from build123d import *

# Parameters (mm, degrees)
F1_DEPTH = 23
F2_DEPTH = 23
F3_DEPTH = 10
F4_R     = 10
F6_D     = 5
F6_DEPTH = 4.3024359474


with BuildPart() as f1:
    # F0 (on Top) → F1 (new body)
    with BuildSketch(Plane.XY):
        with BuildLine():
            ThreePointArc((-10, -72.6985640526), (-1.5147186258, -69.1838454268), (2, -60.6985640526))
            Line((2, -60.6985640526), (2, 4.3014359474))
            Line((2, 4.3014359474), (-28, 4.3014359474))
            Line((-28, 4.3014359474), (-28, -60.6985640526))
            ThreePointArc((-28, -60.6985640526), (-24.4852813742, -69.1838454268), (-16, -72.6985640526))
            Line((-16, -72.6985640526), (-10, -72.6985640526))
        make_face()
        Polygon((-25, -45.6985640526), (-25, -0.6985640526), (-1, -0.6985640526), (-1, -45.6985640526), (0, -45.6985640526), (0, -52.6985640526), (-26, -52.6985640526), (-26, -45.6985640526), align=None, mode=Mode.SUBTRACT)
    extrude(amount=F1_DEPTH)

    # F0 (on Top) → F2 (join)
    with BuildSketch(Plane.XY):
        Polygon((-1, -0.6985640526), (-25, -0.6985640526), (-25, -45.6985640526), (-26, -45.6985640526), (-26, -52.6985640526), (0, -52.6985640526), (0, -45.6985640526), (-1, -45.6985640526), align=None)
    extrude(amount=F2_DEPTH)

    # F0 (on Top) → F3 (cut)
    with BuildSketch(Plane.XY):
        Polygon((-1, -0.6985640526), (-25, -0.6985640526), (-25, -45.6985640526), (-26, -45.6985640526), (-26, -52.6985640526), (0, -52.6985640526), (0, -45.6985640526), (-1, -45.6985640526), align=None)
    extrude(amount=F3_DEPTH, mode=Mode.SUBTRACT)

    # F4
    f4_edges = [f1.edges().sort_by_distance(p)[0] for p in [
        (-28, -28.198564, 23),
    ]]
    fillet(f4_edges, radius=F4_R)

    # F6 (through all, one way)
    with BuildSketch(Plane.XZ):
        with Locations((-13.2052563131, 0)):
            Circle(F6_D / 2)
    extrude(amount=-F6_DEPTH, mode=Mode.SUBTRACT)


solid = f1.part
Input: part model. Units: mm. Frame: model coordinates. A direction names the side the tool comes from. Coordinates: 2 decimals unless noted, no trailing zeros. Order: outer loops, then holes, each group sorted by start corner. A loop starts at its lowest first (then second) coordinate and runs counter-clockwise, first axis right, second up. Notation, with made-up numbers: M 49,0.25 L 63,0.25 A18 cw 63,11.25 Z; hole C -32.5,21 d8. An arc over 180 degrees is marked long. Write item = value, one per line. Start each with the question number.
(1) Reachability of faces 1 (the cylindrical face through (-12.96, -69.85, 19.99)), 2 (the flat face through (-13, -0.699, 5)), 3 (the flat face through (-13, 0, 1)) from +Z, -Z, +X, -X, +Y, -Y: full face, straight path, thin tool, end or side. Return the list, or none.
(2) Section B-B on y = -23. Output: boundary loops of the cut face in (x, z).
(3) Line query: line 1 along X through (y, z) = (-26.5, 3.5); line 2 along Y through (x, z) = (-11.5, 2.25); line 3 along Z through (x, y) = (-12.25, -44). Output: solid intervals per line, ascending. Write a range as [from, to].
(4) Section C-C on z = 12. Output: boundary loops of the cut face in (x, y).
(5) Section D-D on x = -14.75. Output: boundary loops of the cut face in (y, z), and give its area (3 significant figures).
(6) First-contact query: P1, Ø8, axis at x = -17, y = -19, coming from the -Z side; P2, Ø0.8, axis at x = -25.5, z = 3.5, coming from the -Y side; P3, Ø12, axis at y = -63.5, z = 18.5, coming from the -X side. Flat tips, straight axial feed; report the tip coordinate or a pass-through.
(7) Section A-A on z = 7. Output: boundary loops of the cut face in (x, y), and give its area (3 significant figures).
(8) Pull-direction query (X, two-part tool) for faces 4 (the cylindrical face through (-0.85, -27.74, 19.99)), 5 (the flat face through (-25, -23, 5)), 6 (the cylindrical face through (-24.58, -69.09, 6.41)); classes: released by +X, released by -X, zero draft, split by the parting line, or undercut.
Result set:
q1.face_1 = +Z, +X, -X, -Y
q1.face_2 = -Z
q1.face_3 = -Z, +Y
q2.outline = M -28,0 L -25,0 L -25,10 L -1,10 L -1,0 L 2,0 L 2,13 A10 ccw -8,23 L -18,23 A10 ccw -28,13 Z
q3.line_1 = [-28, -25], [-1, 2]
q3.line_2 = [-72.7, -52.7], [-0.7, 4.3]
q3.line_3 = [10, 23]
q4.outline = M -28,-60.7 A12 ccw -16,-72.7 L -10,-72.7 A12 ccw 2,-60.7 L 2,4.3 L -28,4.3 Z
q5.outline = M -72.7,0 L -52.7,0 L -52.7,10 L -0.7,10 L -0.7,0 L 0,0 L 0,1.97 L 4.3,1.97 L 4.3,23 L -62.7,23 A10 ccw -72.7,13 Z
q5.area = 1,220 mm²
q6.P1 = 10
q6.P2 = -68.52
q6.P3 = -28
q7.outline = M -28,-60.7 A12 ccw -16,-72.7 L -10,-72.7 A12 ccw 2,-60.7 L 2,4.3 L -28,4.3 Z; hole M -26,-52.7 L 0,-52.7 L 0,-45.7 L -1,-45.7 L -1,-0.7 L -25,-0.7 L -25,-45.7 L -26,-45.7 Z
q7.area = 986 mm²
q8.face_4 = released by +X
q8.face_5 = undercut
q8.face_6 = released by -X
